```python
from build123d import *

# Parameters (mm, degrees)
SKETCH1_W           = 40
SKETCH1_H           = 40
BOSS_EXTRUDE1_DEPTH = 15
SKETCH2_R           = 1.75
CUT_EXTRUDE1_DEPTH  = 16
SKETCH3_R           = 8.5
CUT_EXTRUDE2_DEPTH  = 41


with BuildPart() as part:
    # Sketch1 → Boss-Extrude1 (new body)
    with BuildSketch(Plane.XY):
        Rectangle(SKETCH1_W, SKETCH1_H)
    extrude(amount=BOSS_EXTRUDE1_DEPTH)

    # Sketch2 → Cut-Extrude1 (cut, through all)
    with BuildSketch(Plane.XY.offset(15)):
        with Locations((-16.5, 0)):
            Circle(SKETCH2_R)
        with Locations((16.5, 0)):
            Circle(SKETCH2_R)
    extrude(amount=-CUT_EXTRUDE1_DEPTH, mode=Mode.SUBTRACT)

    # Sketch3 → Cut-Extrude2 (cut, through all)
    with BuildSketch(Plane(origin=(0, 20, 0), x_dir=(1, 0, 0), z_dir=(0, 1, 0))):
        with Locations((0, -18)):
            Circle(SKETCH3_R)
    extrude(amount=-CUT_EXTRUDE2_DEPTH, mode=Mode.SUBTRACT)


solid = part.part
```
Geometry check sheet. Reference: the model listing, model coordinates, mm. Coordinates: 2 decimals unless noted, no trailing zeros. Order: outer loops, then holes, each group sorted by start corner. A loop starts at its lowest first (then second) coordinate and runs counter-clockwise, first axis right, second up.
Q1. Draft check along X on faces 1 (the face through (20, 0, 7)), 2 (the face through (0, -20, 7)), 3 (the face through (-17.89, -1.06, 7.6)). Enter one of: released by +X, released by -X, zero draft, split by the parting line, or undercut.
Reply:
face 1: released by +X
face 2: zero draft
face 3: undercut
Q2. Sectioned sample at C-C on x = -16.5. Record the cut outline in (y, z), and give its area (4 significant figures).
Reply:
outline: (-20, 0) - (-1.75, 0) - (-1.75, 15) - (-20, 15) - close; (1.75, 0) - (20, 0) - (20, 15) - (1.75, 15) - close
area: 547.5 mm2
Q3. Thickness scan on probe 1 along Y at (x, z) = (-16.5, 3.25); probe 2 along X at (y, z) = (-0.5, 7.25); probe 3 along X at (y, z) = (-1, 1.5). Record the ranges inside material, lowest first.
Reply:
probe 1: y = -20 to -1.75, 1.75 to 20
probe 2: x = -20 to -18.18, -14.82 to 14.82, 18.18 to 20
probe 3: x = -20 to -17.94, -15.06 to 15.06, 17.94 to 20
Q4. Sectioned sample at D-D on z = 13.5. Record the cut outline in (x, y).
Reply:
outline: (-20, -20) - (-7.21, -20) - (-7.21, 20) - (-20, 20) - close; (7.21, -20) - (20, -20) - (20, 20) - (7.21, 20) - close; hole circle Ø3.5 at (-16.5, 0); hole circle Ø3.5 at (16.5, 0)
Q5. Sectioned sample at B-B on y = 0. Record the cut outline in (x, z).
Reply:
outline: (-20, 0) - (-18.25, 0) - (-18.25, 15) - (-20, 15) - close; (-14.75, 0) - (14.75, 0) - (14.75, 15) - (7.95, 15) arc R8.5 cw to (-7.95, 15) - (-14.75, 15) - close; (18.25, 0) - (20, 0) - (20, 15) - (18.25, 15) - close
Q6. Sectioned sample at A-A on z = 10.5. Record the cut outline in (x, y), and give its area (3 significant figures).
Reply:
outline: (-20, -20) - (-4, -20) - (-4, 20) - (-20, 20) - close; (4, -20) - (20, -20) - (20, 20) - (4, 20) - close; hole circle Ø3.5 at (-16.5, 0); hole circle Ø3.5 at (16.5, 0)
area: 1,260 mm2
Q7. Depth check by flat-ended pin: pin 1 Ø3 at (x, y) = (16.5, 0) entering from +Z. Enter the tip coordinate at first touch or a pass-through.
Reply:
pin 1: passes through
